Geometry check sheet. Reference: the model listing, model coordinates, mm. A direction names the side the tool comes from. Round coordinates to 2 decimals unless told otherwise and drop trailing zeros. Order: outer loops, then holes, each group sorted by start corner. A loop starts at its lowest first (then second) coordinate and runs counter-clockwise, first axis right, second up. Notation, with made-up numbers: (24.25, 39) - (75.25, 39) arc R16 cw to (75.25, 66) - close; hole circle Ø3 at (3, 75). An arc over 180 degrees is marked (long way). Use a Markdown table: item, result. Add a question column.
(1) Access from +Z, -Z, +X, -X, +Y, -Y to the whole of each face (thin tool, end or side, straight path). Record for faces 1 (the face through (1, 3.9, -9)), 2 (the face through (6, 8, -1.5)), 3 (the face through (19, 0, -16)), 4 (the face through (-6, 17, 0)).
(2) Section check A-A on x = -9.5. Record the boundary of the cut face in (y, z), then the cut area to 3 significant figures.
(3) Gauge pin test, flat ends, axial feed: P1, Ø4.5, axis at x = -19.45, z = 19.45, coming from the +Y side; P2, Ø1, axis at x = 14.5, z = -8.5, coming from the +Y side; P3, Ø5, axis at x = 4.5, y = 13.5, coming from the +Z side. Record the tip position at first contact, or that the pin passes through.
(4) Section check D-D on z = 27.5. Record the boundary of the cut face in (x, y).
(5) Section check B-B on y = 10.5. Record the boundary of the cut face in (x, z), then the cut area to 3 significant figures.
(6) Thickness scan on line 1 along Z through (x, y) = (-9.5, 2.8); line 2 along X through (y, z) = (-1.3, 0); line 3 along Y through (x, z) = (-1.5, -18). Record the ranges inside material, lowest first. Write a range as [from, to].
(7) Section check C-C on z = 9.5. Record the boundary of the cut face in (x, y).
(8) Mould release check, pull along Z, two halves, no side actions. Record for faces 5 (the face through (-0.88, -1.01, -19.98)), 6 (the face through (-8.428, 9.071, -1.107)), 7 (the face through (0, 3, 14)): released by +Z, released by -Z, zero draft, split by the parting line, or undercut.
```python
from build123d import *

# Parameters (mm, degrees)
HOLE_WIZARD_1_D           = 4
HOLE_WIZARD_1_CSINK_D     = 8
HOLE_WIZARD_1_CSINK_ANGLE = 90
CUT_EXTRUDE_1_DEPTH       = 48.716978111
SKETCH_12_R               = 8.5
EXTRUDE_1_DEPTH           = 1.9
FILLET_2_R                = 0.15
CHAMFER_3_SIZE            = 0.5
HOLE_WIZARD_M2_1_D        = 1.6
SKETCH_11_R               = 4
CUT_EXTRUDE_2_DEPTH       = 47.695824224


with BuildPart() as part:
    # 草图1 → 旋转1 (revolve)
    with BuildSketch(Plane.XY, mode=Mode.PRIVATE) as revolve_1_sk:
        Polygon((24.5, 0), (31.5, 0), (31.5, 3), (11.5, 3), (11.5, 3.9), (8.5, 3.9), (8.5, 14.1), (8, 14.1), (8, 15.1), (5, 15.1), (5, 0), (20, 0), (20, -2), (24.5, -2), align=None)
    revolve(revolve_1_sk.sketch.rotate(Axis((0, 57.09591982, 0), (0, -1, 0)), 90), axis=Axis((0, 57.09591982, 0), (0, -1, 0)))

    # 打孔尺寸(%根据十字)槽半沉头木螺钉的类型1 (through all)
    with Locations(Plane(origin=(0, 3, 0), x_dir=(-1, 0, 0), z_dir=(0, 1, 0))):
        with Locations((0, 27.5), (-19.445436483, -19.445436483), (-27.5, 0), (-19.445436483, 19.445436483), (0, -27.5), (19.445436483, -19.445436483), (27.5, 0), (19.445436483, 19.445436483)):
            CounterSinkHole(HOLE_WIZARD_1_D / 2, HOLE_WIZARD_1_CSINK_D / 2, counter_sink_angle=HOLE_WIZARD_1_CSINK_ANGLE)

    # 草图7 → 切除-拉伸1 (cut, through all)
    with BuildSketch(Plane(origin=(0, 15.1, 0), x_dir=(1, 0, 0), z_dir=(0, 1, 0))):
        with BuildLine():
            Line((6.4, -1.5), (6.4, 1.5))
            Line((6.4, 1.5), (4.769696007, 1.5))
            ThreePointArc((4.769696007, 1.5), (5, 0), (4.769696007, -1.5))
            Line((4.769696007, -1.5), (6.4, -1.5))
        make_face()
    extrude(amount=-CUT_EXTRUDE_1_DEPTH, mode=Mode.SUBTRACT)

    # 草图12 → 凸台-拉伸1 (add)
    with BuildSketch(Plane(origin=(0, 15.1, 0), x_dir=(1, 0, 0), z_dir=(0, 1, 0))):
        with Locations(Location((0, 0, 0), (0, 0, 270))):
            Circle(SKETCH_12_R)
        with BuildLine():
            Line((6.4, 1.5), (4.769696007, 1.5))
            ThreePointArc((4.769696007, 1.5), (-5, 0), (4.769696007, -1.5))
            Line((4.769696007, -1.5), (6.4, -1.5))
            Line((6.4, -1.5), (6.4, 1.5))
        make_face(mode=Mode.SUBTRACT)
    extrude(amount=EXTRUDE_1_DEPTH)

    # 圆角2
    fillet_2_edges = [part.edges().sort_by_distance(p)[0] for p in [
        (6.4, 7.55, -1.5),
        (6.4, 7.55, 1.5),
    ]]
    fillet(fillet_2_edges, radius=FILLET_2_R)

    # 倒角3
    chamfer_3_edges = [part.edges().sort_by_distance(p)[0] for p in [
        (-5, 17, 0),
        (-5, 0, 0),
    ]]
    chamfer(chamfer_3_edges, length=CHAMFER_3_SIZE)

    # M2 螺纹孔1 (through all)
    with Locations(Plane(origin=(0, 3.9, 0), x_dir=(1, 0, 0), z_dir=(0, 1, 0))):
        with Locations((9.5, 0), (0, -9.5), (0, 9.5), (-9.5, 0)):
            Hole(HOLE_WIZARD_M2_1_D / 2)

    # 草图11 → 切除-拉伸2 (cut, through all)
    with BuildSketch(Plane(origin=(0, 3, 0), x_dir=(1, 0, 0), z_dir=(0, 1, 0))):
        with Locations(Location((11.313708499, 11.313708499, 0), (0, 0, 270))):
            Circle(SKETCH_11_R)
        with Locations(Location((11.313708499, -11.313708499, 0), (0, 0, 270))):
            Circle(SKETCH_11_R)
        with Locations(Location((-11.313708499, -11.313708499, 0), (0, 0, 270))):
            Circle(SKETCH_11_R)
        with Locations(Location((-11.313708499, 11.313708499, 0), (0, 0, 270))):
            Circle(SKETCH_11_R)
    extrude(amount=-CUT_EXTRUDE_2_DEPTH, mode=Mode.SUBTRACT)


solid = part.part
```
Check sheet entries:
| question | item | result |
|---|---|---|
| 1 | face 1 | +Y |
| 1 | face 2 | +Y, -Y |
| 1 | face 3 | -Y |
| 1 | face 4 | +Z, -Z, +X, -X, +Y |
| 2 | outline | (-2, -22.58) - (0, -22.58) - (0, -30.03) - (3, -30.03) - (3, -14.88) - (0, -14.88) - (0, -17.6) - (-2, -17.6) - close; (-2, 17.6) - (0, 17.6) - (0, 14.88) - (3, 14.88) - (3, 30.03) - (0, 30.03) - (0, 22.58) - (-2, 22.58) - close; (0, -7.75) - (3, -7.75) - (3, -6.48) - (3.9, -6.48) - (3.9, -0.8) - (0, -0.8) - close; (0, 0.8) - (3.9, 0.8) - (3.9, 6.48) - (3, 6.48) - (3, 7.75) - (0, 7.75) - close |
| 2 | area | 163 mm2 |
| 3 | P1 | stops at y = 1.26 |
| 3 | P2 | stops at y = 3 |
| 3 | P3 | stops at z = 8.26 |
| 4 | outline | (-15.36, 0) - (-2, 0) - (-2, 1) - (-4, 3) - (-15.36, 3) - close; (2, 0) - (15.36, 0) - (15.36, 3) - (4, 3) - (2, 1) - close |
| 5 | outline | circle Ø17 at (0, 0); hole (4.77, -1.5) - (6.25, -1.5) arc R0.15 ccw to (6.4, -1.35) - (6.4, 1.35) arc R0.15 ccw to (6.25, 1.5) - (4.77, 1.5) arc R5 ccw (long way) to start |
| 5 | area | 144 mm2 |
| 6 | line 1 | z = [-30.03, -14.88], [-7.75, -0.8], [0.8, 7.75], [14.88, 30.03] |
| 6 | line 2 | x = [-24.5, -20], [20, 24.5] |
| 6 | line 3 | y = [0, 3] |
| 7 | outline | (-30.03, 0) - (-22.58, 0) - (-22.58, -2) - (-17.6, -2) - (-17.6, 0) - (-14.88, 0) - (-14.88, 3) - (-30.03, 3) - close; (-7.75, 0) - (-0.8, 0) - (-0.8, 3.9) - (-6.48, 3.9) - (-6.48, 3) - (-7.75, 3) - close; (0.8, 0) - (7.75, 0) - (7.75, 3) - (6.48, 3) - (6.48, 3.9) - (0.8, 3.9) - close; (14.88, 0) - (17.6, 0) - (17.6, -2) - (22.58, -2) - (22.58, 0) - (30.03, 0) - (30.03, 3) - (14.88, 3) - close |
| 8 | face 5 | undercut |
| 8 | face 6 | split by the parting line |
| 8 | face 7 | zero draft |
